The listing builds one solid part. Answer for the finished solid, in the listing's coordinates (mm). A direction names the side the tool comes from. Round coordinates to 2 decimals unless told otherwise and drop trailing zeros. Write each loop counter-clockwise with the first axis right and the second up, starting at its lowest first coordinate (ties: lowest second). Pieces come first, ordered by that corner, then holes. Notation, with made-up numbers: M 26.5,87.25 L 67.5,87.25 A25 cw 67.5,110.25 Z; hole C 13.25,39.25 d4. An arc over 180 degrees is marked long. One line per item, written item: value. Start each with the question number.
(1) Given P1, Ø1, axis at y = 3.5, z = -3, coming from the -X side; P2, Ø1.5, axis at y = 1, z = -5, coming from the -X side, each flat-ended and moving along its own axis, determine where each tip first touches the part or whether it passes through.
(2) For faces 4 (the flat face through (8, 0, 0)), 5 (the flat face through (20, 2, 2.05)), determine the directions among +Z, -Z, +X, -X, +Y, -Y from which every point of the face is accessible in a straight line to the end or side of a thin tool.
(3) Section A-A (x = 19) is taken. Determine the outline of the cut face in (y, z), plus the area to 3 significant figures.
(4) Section D-D (z = 6) is taken. Determine the outline of the cut face in (x, y), plus the area to 3 significant figures.
(5) Consider probe 1 along X at (y, z) = (1.95, 0); probe 2 along Z at (x, y) = (21, 2.1); probe 3 along X at (y, z) = (1.4, -1.25). Determine where each line is inside the solid, lowest interval first.
(6) Section C-C (y = 2.6) is taken. Determine the outline of the cut face in (x, z), plus the area to 3 significant figures.
(7) Section B-B (z = 0) is taken. Determine the outline of the cut face in (x, y).
(8) For a pull along Z with two mould halves and no side action, classify faces 1 (the cylindrical face through (27.759, 1.972, 2.335)), 2 (the cylindrical face through (27.775, 1.972, 9.199)), 3 (the flat face through (28.06, 2, -6)) as released by +Z, released by -Z, zero draft, split by the parting line, or undercut.
```python
from build123d import *

# Parameters (mm, degrees)
SKETCH1_R           = 2.55
BOSS_EXTRUDE1_DEPTH = 4


with BuildPart() as part:
    # Sketch1 → Boss-Extrude1 (new body)
    with BuildSketch(Plane(origin=(0, 0, 0), x_dir=(1, 0, 0), z_dir=(0, 1, 0))):
        with BuildLine():
            Line((27.06, 2.05), (12.15, 2.05))
            Line((12.15, 2.05), (12.15, -2.05))
            Line((12.15, -2.05), (27.06, -2.05))
            ThreePointArc((27.06, -2.05), (27.767106781, -2.342893219), (28.06, -3.05))
            Line((28.06, -3.05), (28.06, -8.5))
            ThreePointArc((28.06, -8.5), (27.767106781, -9.207106781), (27.06, -9.5))
            Line((27.06, -9.5), (-2.15, -9.5))
            ThreePointArc((-2.15, -9.5), (-11.65, 0), (-2.15, 9.5))
            Line((-2.15, 9.5), (27.06, 9.5))
            ThreePointArc((27.06, 9.5), (27.767106781, 9.207106781), (28.06, 8.5))
            Line((28.06, 8.5), (28.06, 3.05))
            ThreePointArc((28.06, 3.05), (27.767106781, 2.342893219), (27.06, 2.05))
        make_face()
        with Locations(Location((-2.15, 0, 0), (0, 0, 270))):
            Circle(SKETCH1_R, mode=Mode.SUBTRACT)
    extrude(amount=BOSS_EXTRUDE1_DEPTH)


solid = part.part
```
Recorded:
1. P1: stops at x = -11.32
1. P2: stops at x = -10.65
2. face 4: +Z, -Z, +X, -X, -Y
2. face 5: +X, +Y, -Y
3. outline: M 0,-9.5 L 4,-9.5 L 4,-2.05 L 0,-2.05 Z; M 0,2.05 L 4,2.05 L 4,9.5 L 0,9.5 Z
3. area: 59.6 mm2
4. outline: M -9.52,0 L 28.06,0 L 28.06,4 L -9.52,4 Z
4. area: 150 mm2
5. probe 1: x = -11.65 to -4.7, 0.4 to 12.15
5. probe 2: z = -9.5 to -2.05, 2.05 to 9.5
5. probe 3: x = -11.57 to -4.37, 0.07 to 12.15
6. outline: M -2.15,-9.5 L 27.06,-9.5 A1 ccw 28.06,-8.5 L 28.06,-3.05 A1 ccw 27.06,-2.05 L 12.15,-2.05 L 12.15,2.05 L 27.06,2.05 A1 ccw 28.06,3.05 L 28.06,8.5 A1 ccw 27.06,9.5 L -2.15,9.5 A9.5 ccw Z; hole C -2.15,0 d5.1
6. area: 629 mm2
7. outline: M -11.65,0 L -4.7,0 L -4.7,4 L -11.65,4 Z; M 0.4,0 L 12.15,0 L 12.15,4 L 0.4,4 Z
8. face 1: undercut
8. face 2: released by +Z
8. face 3: zero draft
